```python
from build123d import *

# Parameters (mm, degrees)
PAD021_DEPTH                        = 3
SKETCH083_R                         = 1.7
POCKET041_DEPTH                     = 0.001
POCKET041_DEPTH_BACK                = 3.001
SKETCH084_R                         = 1.7
POCKET042_DEPTH                     = 0.001
POCKET042_DEPTH_BACK                = 3.001
BODY001003005003013_PLACEMENT_ANGLE = 60


with BuildPart() as part:
    # Sketch082 → Pad021 (new body)
    with BuildSketch(Plane.XY):
        with BuildLine():
            ThreePointArc((156.715765, 119.164267), (87.462654, 176.380945), (0, 196.875477))
            Line((0, 196.875477), (0, 181.875477))
            ThreePointArc((144.775545, 110.085106), (80.798849, 162.942429), (0, 181.875477))
            ThreePointArc((148.119912, 105.542318), (146.465342, 107.826679), (144.775545, 110.085106))
            ThreePointArc((148.119912, 105.542318), (148.721895, 105.145439), (149.434315, 105.256592))
            Line((155.166125, 108.565855), (149.434315, 105.256592))
            Line((155.166125, 108.565855), (160.740736, 111.784358))
            ThreePointArc((160.740736, 111.784358), (161.217235, 112.43486), (161.058811, 113.225496))
            ThreePointArc((161.058811, 113.225496), (158.915032, 116.215171), (156.715765, 119.164267))
        make_face()
    pad021 = extrude(amount=PAD021_DEPTH)

    # Mirrored029: Pad021 across Sketch082 V_Axis
    add(pad021.mirror(Plane(origin=(0, 0, 0), x_dir=(0, 0, 1), z_dir=(1, 0, 0))))

    # Sketch083 → Pocket041 (cut, two sides)
    with BuildSketch(Plane.XY) as pocket041_sk:
        with Locations((149.218956, 116.605208)):
            Circle(SKETCH083_R)
        with Locations((-149.218956, 116.605208)):
            Circle(SKETCH083_R)
    extrude(amount=-POCKET041_DEPTH, mode=Mode.SUBTRACT)
    extrude(pocket041_sk.sketch, amount=POCKET041_DEPTH_BACK, mode=Mode.SUBTRACT)

    # Sketch084 → Pocket042 (cut, two sides)
    with BuildSketch(Plane.XY) as pocket042_sk:
        with Locations((0, 189.375477)):
            Circle(SKETCH084_R)
    extrude(amount=-POCKET042_DEPTH, mode=Mode.SUBTRACT)
    extrude(pocket042_sk.sketch, amount=POCKET042_DEPTH_BACK, mode=Mode.SUBTRACT)


with BuildPart() as part_1:
    # Body001003005003013 placement: moved
    add(part.part.rotate(Axis((0, 0, 0), (0, 0, 1)), BODY001003005003013_PLACEMENT_ANGLE))


solid = part_1.part
```
Input: part model. Units: mm. Frame: model coordinates. Round coordinates to 2 decimals unless told otherwise and drop trailing zeros. Order: outer loops, then holes, each group sorted by start corner. A loop starts at its lowest first (then second) coordinate and runs counter-clockwise, first axis right, second up. Notation, with made-up numbers: (1.5, 34.25) - (53.5, 34.25) arc R17 cw to (53.5, 45.25) - close; hole circle Ø6 at (88, 10). An arc over 180 degrees is marked (long way). One line per question, with ' | ' between items. Start each with the question number.
1) Contact query for a flat-ended pin moving along its axis: P1, Ø2.5, axis at x = -175.59, y = -70.92, coming from the +Z side. Output: stop coordinate, or through.
2) Cut plane B-B, the plane x = -153. Return the cut outline in (y, z), then the cut area to 3 significant figures.
3) Cut plane C-C, the plane y = 139. Return the cut outline in (x, z), then the cut area to 3 significant figures.
4) Cut plane A-A, the plane z = 1.1. Return the cut outline in (x, y).
5) Ray query, probe 1 along Y at (x, z) = (-167.5, 2.55); probe 2 along Y at (x, z) = (-25, 1.8); probe 3 along Y at (x, z) = (-122.5, 2.65). Return the intervals inside material, ascending.
Worked out:
1) P1: passes through
2) outline: (98.33, 0) - (123.9, 0) - (123.9, 3) - (98.33, 3) - close | area: 76.7 mm^2
3) outline: (-139.42, 0) - (-117.29, 0) - (-117.29, 3) - (-139.42, 3) - close | area: 66.4 mm^2
4) outline: (-181.56, -76.14) arc R196.88 ccw to (-178.59, -82.87) arc R1 ccw to (-177.18, -83.31) - (-171.6, -80.09) - (-165.87, -76.79) arc R1 ccw to (-165.46, -75.5) arc R181.88 cw to (-167.72, -70.34) arc R181.88 cw to (-157.51, 90.94) arc R181.88 cw to (-22.95, 180.42) arc R181.88 cw to (-17.34, 181.05) arc R1 ccw to (-16.44, 182.04) - (-16.44, 188.66) - (-16.44, 195.1) arc R1 ccw to (-17.53, 196.09) arc R196.88 ccw to (-24.84, 195.3) arc R196.88 ccw to (-170.5, 98.44) arc R196.88 ccw to start; hole circle Ø3.4 at (-175.59, -70.92); hole circle Ø3.4 at (-164, 94.69); hole circle Ø3.4 at (-26.37, 187.53)
5) probe 1: y = -77.73 to -70.87, 70.87 to 103.46 | probe 2: y = 180.15 to 186.53, 188.53 to 195.28 | probe 3: y = 134.43 to 154.12
